Geometry: final body of the model. Coordinates: model frame, mm. A direction names the side the tool comes from. Coordinates: 2 decimals unless noted, no trailing zeros. Write each loop counter-clockwise with the first axis right and the second up, starting at its lowest first coordinate (ties: lowest second). Pieces come first, ordered by that corner, then holes. Notation, with made-up numbers: (-11.75, 89.25) -> (46.25, 89.25) arc R25 cw to (46.25, 101.25) -> close; hole circle Ø2 at (14.25, 53). An arc over 180 degrees is marked (long way). Answer as a JSON object with one key per item and string values. Group by question number.
```python
from build123d import *

# Parameters (mm, degrees)
PAD132_DEPTH    = 20
SKETCH277_W     = 18
SKETCH277_H     = 5
POCKET115_DEPTH = 20
SKETCH278_W     = 34
SKETCH278_H     = 18
PAD133_DEPTH    = 2
SKETCH279_W     = 61
SKETCH279_H     = 49.5
SKETCH279_W_2   = 31
SKETCH279_H_2   = 15
POCKET116_DEPTH = 18
SKETCH280_R     = 2.25
POCKET117_DEPTH = 5
SKETCH281_W     = 3
SKETCH281_H     = 11
POCKET118_DEPTH = 8


with BuildPart() as part:
    # Sketch276 → Pad132 (new body)
    with BuildSketch(Plane.XY):
        with BuildLine():
            Line((-16, 7.96043), (16, 7.96043))
            Line((16, 7.96043), (23.820487, 9.858884))
            ThreePointArc((26.179513, 0.141116), (29.858884, 6.179513), (23.820487, 9.858884))
            Line((16, -2.33), (26.179513, 0.141116))
            Line((16, -2.33), (16, -8.03957))
            Line((16, -8.03957), (3.900743, -23.127972))
            ThreePointArc((-3.900743, -23.127972), (0, -25), (3.900743, -23.127972))
            Line((-16, -8.03957), (-3.900743, -23.127972))
            Line((-16, -8.03957), (-16, -2.33))
            Line((-16, -2.33), (-26.179513, 0.141116))
            ThreePointArc((-23.820487, 9.858884), (-29.858884, 6.179513), (-26.179513, 0.141116))
            Line((-16, 7.96043), (-23.820487, 9.858884))
        make_face()
        Polygon((-14, 6.5), (-14, 0), (-12.5, 0), (-12.5, -6.5), (-11, -6.5), (-11, 0), (11, 0), (11, -6.5), (12.5, -6.5), (12.5, 0), (14, 0), (14, 6.5), align=None, mode=Mode.SUBTRACT)
        with BuildLine():
            ThreePointArc((4.26793, -17.39524), (0, -15), (-4.26793, -17.39524))
            Line((-11, -9), (-4.26793, -17.39524))
            Line((-11, -9), (11, -9))
            Line((11, -9), (4.26793, -17.39524))
        make_face(mode=Mode.SUBTRACT)
    extrude(amount=PAD132_DEPTH)

    # Sketch277 (on Face29 of Pad132) → Pocket115 (cut)
    with BuildSketch(Plane(origin=(0, 0, 0), x_dir=(1, 0, 0), z_dir=(0, 0, -1))):
        with Locations((0, 3.5)):
            Rectangle(SKETCH277_W, SKETCH277_H)
    extrude(amount=-POCKET115_DEPTH, mode=Mode.SUBTRACT)

    # Sketch278 (on Face4 of Pocket115) → Pad133 (join)
    with BuildSketch(Plane(origin=(0, 0, 0), x_dir=(1, 0, 0), z_dir=(0, 0, -1))):
        Rectangle(SKETCH278_W, SKETCH278_H)
    extrude(amount=-PAD133_DEPTH)

    # Sketch279 (on Face32 of Pad133) → Pocket116 (cut, symmetric)
    with BuildSketch(Plane.XY.offset(20)):
        with Locations((0, -4.75)):
            Rectangle(SKETCH279_W, SKETCH279_H)
        Rectangle(SKETCH279_W_2, SKETCH279_H_2, mode=Mode.SUBTRACT)
    extrude(amount=POCKET116_DEPTH, both=True, mode=Mode.SUBTRACT)

    # Sketch280 → Pocket117 (cut)
    with BuildSketch(Plane.XY):
        with Locations((0, -20)):
            Circle(SKETCH280_R)
        with Locations((25, 5)):
            Circle(SKETCH280_R)
        with Locations((-25, 5)):
            Circle(SKETCH280_R)
    extrude(amount=POCKET117_DEPTH, mode=Mode.SUBTRACT)

    # Sketch281 (on Face37 of Pocket117) → Pocket118 (cut)
    with BuildSketch(Plane.XZ.offset(7.5)):
        with Locations((-11.75, 10.5)):
            Rectangle(SKETCH281_W, SKETCH281_H)
        with Locations((11.75, 10.5)):
            Rectangle(SKETCH281_W, SKETCH281_H)
    extrude(amount=-POCKET118_DEPTH, mode=Mode.SUBTRACT)


with BuildPart() as part_1:
    # Body030 placement: moved
    add(part.part.moved(Location((0, 0, -33))))


solid = part_1.part
```
Item 1: Section C-C on y = 5. Output: boundary loops of the cut face in (x, z), then the cut area to 3 significant figures.
Item 2: Mould query, pull axis Z, two halves, no side actions, for faces 1 (the flat face through (12.5, -3, -30)), 2 (the flat face through (0, -4, -31)), 3 (the flat face through (13.25, -4, -23)), 4 (the flat face through (-10.25, -4, -23)). Classes: +Z half, -Z half, draft (parallel to the pull), parting line (faces both ways), or undercut.
Item 3: Contact query for flat-ended pins moving along their axis: pin 1 (12 mm diameter, centred on x = 8, y = -17, fed in from +Z); pin 2 (1 mm diameter, centred on x = 12.5, z = -29.5, fed in from +Y); pin 3 (1 mm diameter, centred on x = -3, z = -32.5, fed in from -Y); pin 4 (2.5 mm diameter, centred on x = -11.5, y = -2, fed in from +Z). Output: stop coordinate, or through.
Item 4: Set-up query: faces 5 (the flat face through (-16, -9, -32)), 6 (the flat face through (0, 0, -22)), 7 (the flat face through (-7.68, -13.14, -32.01)). Return all of +Z, -Z, +X, -X, +Y, -Y with unobstructed straight access to the full face (end or side cutting, diameter ignored); none if empty.
Item 5: Section B-B on x = 0. Output: boundary loops of the cut face in (y, z).
Item 6: Section A-A on z = -17.75. Output: boundary loops of the cut face in (x, y), then the cut area to 3 significant figures.
Item 7: Section D-D on z = -14.75. Output: boundary loops of the cut face in (x, y), then the cut area to 4 significant figures.
Item 8: Ray query, L1, parallel to X at y = -0.5, z = -14; L2, parallel to X at y = 5, z = -32.1; L3, parallel to X at y = -2, z = -25. Return the intervals inside material, ascending. Write a range as [from, to].
Answer sheet:
{
 "1": {"outline": "(-30, -33) -> (-27.25, -33) -> (-27.25, -31) -> (-30, -31) -> close; (-22.75, -33) -> (22.75, -33) -> (22.75, -31) -> (15.5, -31) -> (15.5, -13) -> (14, -13) -> (14, -31) -> (-14, -31) -> (-14, -13) -> (-15.5, -13) -> (-15.5, -31) -> (-22.75, -31) -> close; (27.25, -33) -> (30, -33) -> (30, -31) -> (27.25, -31) -> close", "area": "156 mm^2"},
 "2": {"face 1": "draft", "face 2": "+Z half", "face 3": "undercut", "face 4": "undercut"},
 "3": {"pin 1": "stops at z = -31", "pin 2": "stops at y = 7.5", "pin 3": "stops at y = -24.33", "pin 4": "stops at z = -13"},
 "4": {"face 5": "+Z, -Z, -X, -Y", "face 6": "+Z", "face 7": "+Z, -Z"},
 "5": {"outline": "(-25, -33) -> (-22.25, -33) -> (-22.25, -31) -> (-25, -31) -> close; (-17.75, -33) -> (-15, -33) -> (-15, -31) -> (-17.75, -31) -> close; (-9, -33) -> (9, -33) -> (9, -31) -> (7.5, -31) -> (7.5, -13) -> (6.5, -13) -> (6.5, -31) -> (0, -31) -> (0, -13) -> (-1, -13) -> (-1, -31) -> (-6, -31) -> (-6, -13) -> (-7.5, -13) -> (-7.5, -31) -> (-9, -31) -> close"},
 "6": {"outline": "(-15.5, -7.5) -> (-13.25, -7.5) -> (-13.25, 0) -> (-14, 0) -> (-14, 6.5) -> (14, 6.5) -> (14, 0) -> (13.25, 0) -> (13.25, -7.5) -> (15.5, -7.5) -> (15.5, 7.5) -> (-15.5, 7.5) -> close; (-10.25, -7.5) -> (10.25, -7.5) -> (10.25, 0) -> (-10.25, 0) -> close; hole (-9, -6) -> (9, -6) -> (9, -1) -> (-9, -1) -> close", "area": "148 mm^2"},
 "7": {"outline": "(-15.5, -7.5) -> (15.5, -7.5) -> (15.5, 7.5) -> (-15.5, 7.5) -> close; hole (-14, 0) -> (-12.5, 0) -> (-12.5, -6.5) -> (-11, -6.5) -> (-11, 0) -> (11, 0) -> (11, -6.5) -> (12.5, -6.5) -> (12.5, 0) -> (14, 0) -> (14, 6.5) -> (-14, 6.5) -> close; hole (-9, -6) -> (9, -6) -> (9, -1) -> (-9, -1) -> close", "area": "173.5 mm^2"},
 "8": {"L1": "x = [-15.5, -12.5], [-11, 11], [12.5, 15.5]", "L2": "x = [-30, -27.25], [-22.75, 22.75], [27.25, 30]", "L3": "x = [-15.5, -13.25], [-10.25, -9], [9, 10.25], [13.25, 15.5]"}
}
